Input: part model. Units: mm. Frame: model coordinates. Round coordinates to 2 decimals unless told otherwise and drop trailing zeros. Loops run counter-clockwise (first coordinate to the right, second up) from the corner with the lowest first, then second, coordinate; pieces in that order, holes last. Notation, with made-up numbers: (-1, 84.5) - (42, 84.5) arc R7 ccw to (42, 92.5) - close; hole circle Ø6 at (10, 51). An arc over 180 degrees is marked (long way). Write each question's results on one line, items separated by ' | '.
from build123d import *

# Parameters (mm, degrees)
F1_DEPTH    = 3
F2_DEPTH    = 25
F3_R        = 20
F4_R        = 100
F5_T1_DEPTH = 28.2643660281


# Not quite as in the source:
# - a fillet or chamfer that OpenCascade refuses, or shapes differently, is made with other operations: its cross-section is extruded or revolved along the edge and cut away or added


with BuildPart() as f1:
    # F0 (on Front) → F1 (new body)
    with BuildSketch(Plane.XZ):
        with BuildLine():
            ThreePointArc((-119.2295857728, 16.5976797057), (-89.2269882152, -21.8866064143), (-44.5863344816, -2.1785326218))
            ThreePointArc((-44.5863344816, -2.1785326218), (-31.5003837254, 22.7075657451), (-18.8527258188, 47.819251244))
            ThreePointArc((-18.8527258188, 47.819251244), (-11.5073907558, 58.7139707042), (-8.9261215756, 71.5975225718))
            Line((-8.9261215756, 71.5975225718), (-11.67442069, 71.5975225718))
            Line((-11.67442069, 71.5975225718), (-11.67442069, 74.0203762137))
            ThreePointArc((-11.67442069, 74.0203762137), (-12.7707106261, 77.9833199576), (-14.3762885703, 81.7686725444))
            ThreePointArc((-14.3762885703, 81.7686725444), (-44.33377908, 98.9465167224), (-71.9061774941, 78.1548738354))
            Line((-71.9061774941, 78.1548738354), (-107.2845857728, 78.1548738354))
            Line((-107.2845857728, 78.1548738354), (-119.2295857728, 78.1548738354))
            Line((-119.2295857728, 78.1548738354), (-119.2295857728, 66.2098738354))
            Line((-119.2295857728, 66.2098738354), (-119.2295857728, 16.5976797057))
        make_face()
        with BuildLine():
            ThreePointArc((-26.6928125913, 79.0930187933), (-24.6315082315, 75.5227380173), (-23.3711215756, 71.597523888))
            Line((-23.3711215756, 71.597523888), (-20.8711215756, 71.5975236602))
            ThreePointArc((-20.8711215756, 71.5975236602), (-22.8939959961, 62.4935676044), (-28.5819229469, 55.1029300277))
            ThreePointArc((-28.5819229469, 55.1029300277), (-41.6104278008, 29.1671780434), (-55.1096433175, 3.4732809051))
            ThreePointArc((-55.1096433175, 3.4732809051), (-86.3130475025, -10.3024804429), (-107.2845857728, 16.5976797057))
            Line((-107.2845857728, 16.5976797057), (-107.2845857728, 66.2098738354))
            Line((-107.2845857728, 66.2098738354), (-104.7845857728, 66.2098738354))
            Line((-104.7845857728, 66.2098738354), (-68.5864427672, 66.2098738354))
            Line((-68.5864427672, 66.2098738354), (-63.1803487139, 66.2098738354))
            ThreePointArc((-63.1803487139, 66.2098738354), (-63.6941147242, 68.8812286524), (-63.8664115811, 71.5960777945))
            Line((-63.8664115811, 71.5960777945), (-61.3664115868, 71.5962461647))
            ThreePointArc((-61.3664115868, 71.5962461647), (-46.4685424734, 86.625019162), (-26.6928125913, 79.0930187933))
        make_face(mode=Mode.SUBTRACT)
        with BuildLine():
            ThreePointArc((-32.7025071715, 52.3956462756), (-51.243606048, 52.0172813271), (-63.1803487139, 66.2098738354))
            Line((-63.1803487139, 66.2098738354), (-68.5864427672, 66.2098738354))
            Line((-68.5864427672, 66.2098738354), (-104.7845857728, 66.2098738354))
            Line((-104.7845857728, 66.2098738354), (-104.7845857728, 16.5976797057))
            ThreePointArc((-104.7845857728, 16.5976797057), (-85.7031813006, -7.8780087034), (-57.3120938901, 4.6561636023))
            ThreePointArc((-57.3120938901, 4.6561636023), (-44.8056231456, 28.4219407394), (-32.7025071715, 52.3956462756))
        make_face()
        with BuildLine():
            ThreePointArc((-61.3664115868, 71.5962461647), (-42.368127741, 52.5998806027), (-23.3711215756, 71.597523888))
            Line((-23.3711215756, 71.597523888), (-28.5062876117, 71.7030383349))
            ThreePointArc((-28.5062876117, 71.7030383348), (-35.0280474509, 67.9936357913), (-42.4162418184, 66.6868830916))
            ThreePointArc((-42.4162418184, 66.6868830916), (-49.8149115034, 67.9342855665), (-56.3664115866, 71.5913571683))
            Line((-56.3664115866, 71.5913571683), (-61.3664115868, 71.5962461647))
        make_face()
        with BuildLine():
            ThreePointArc((-55.1096433175, 3.4732809051), (-41.6104278008, 29.1671780434), (-28.5819229469, 55.1029300277))
            ThreePointArc((-28.5819229469, 55.1029300277), (-30.5643455059, 53.6307678626), (-32.7025071715, 52.3956462756))
            ThreePointArc((-32.7025071715, 52.3956462756), (-44.8056231456, 28.4219407394), (-57.3120938901, 4.6561636023))
            ThreePointArc((-57.3120938901, 4.6561636023), (-85.7031813006, -7.8780087034), (-104.7845857728, 16.5976797057))
            Line((-104.7845857728, 16.5976797057), (-104.7845857728, 66.2098738354))
            Line((-104.7845857728, 66.2098738354), (-107.2845857728, 66.2098738354))
            Line((-107.2845857728, 66.2098738354), (-107.2845857728, 16.5976797057))
            ThreePointArc((-107.2845857728, 16.5976797057), (-86.3130475025, -10.3024804429), (-55.1096433175, 3.4732809051))
        make_face()
        with BuildLine():
            ThreePointArc((-42.4162418184, 66.6868830916), (-35.0280474509, 67.9936357913), (-28.5062876117, 71.7030383348))
            ThreePointArc((-28.5062876117, 71.7030383349), (-42.4756351565, 81.447422187), (-56.3664115866, 71.5913571683))
            ThreePointArc((-56.3664115866, 71.5913571683), (-49.8149115034, 67.9342855665), (-42.4162418184, 66.6868830916))
        make_face()
        with BuildLine():
            Line((-28.5062876117, 71.7030383349), (-23.3711215756, 71.597523888))
            ThreePointArc((-23.3711215756, 71.597523888), (-24.6315082315, 75.5227380173), (-26.6928125913, 79.0930187933))
            ThreePointArc((-26.6928125913, 79.0930187933), (-46.4685424734, 86.625019162), (-61.3664115868, 71.5962461647))
            Line((-61.3664115868, 71.5962461647), (-56.3664115866, 71.5913571683))
            ThreePointArc((-56.3664115866, 71.5913571683), (-42.4756351565, 81.447422187), (-28.5062876117, 71.7030383349))
        make_face()
        with BuildLine():
            Line((-20.8711215756, 71.5975236602), (-23.3711215756, 71.597523888))
            ThreePointArc((-23.3711215756, 71.597523888), (-42.368127741, 52.5998806027), (-61.3664115868, 71.5962461647))
            Line((-61.3664115868, 71.5962461647), (-63.8664115811, 71.5960777945))
            ThreePointArc((-63.8664115811, 71.5960777945), (-63.6941147242, 68.8812286524), (-63.1803487139, 66.2098738354))
            ThreePointArc((-63.1803487139, 66.2098738354), (-51.243606048, 52.0172813271), (-32.7025071715, 52.3956462756))
            ThreePointArc((-32.7025071715, 52.3956462756), (-30.5643455059, 53.6307678626), (-28.5819229469, 55.1029300277))
            ThreePointArc((-28.5819229469, 55.1029300277), (-22.8939959961, 62.4935676044), (-20.8711215756, 71.5975236602))
        make_face()
    extrude(amount=F1_DEPTH)

    # F0 (on Front) → F2 (cut)
    with BuildSketch(Plane.XZ):
        with BuildLine():
            ThreePointArc((-42.4162418184, 66.6868830916), (-35.0280474509, 67.9936357913), (-28.5062876117, 71.7030383348))
            ThreePointArc((-28.5062876117, 71.7030383349), (-42.4756351565, 81.447422187), (-56.3664115866, 71.5913571683))
            ThreePointArc((-56.3664115866, 71.5913571683), (-49.8149115034, 67.9342855665), (-42.4162418184, 66.6868830916))
        make_face()
    extrude(amount=F2_DEPTH, mode=Mode.SUBTRACT)

    # F3
    f3_edges = [f1.edges().sort_by_distance(p)[0] for p in [
        (-119.229586, -1.5, 78.154874),
    ]]
    fillet(f3_edges, radius=F3_R)

    # F4
    f4_edges = [f1.edges().sort_by_distance(p)[0] for p in [
        (-71.906177, -1.5, 78.154874),
    ]]
    fillet(f4_edges, radius=F4_R)

    # F5: fillet of radius 5 on 1 edges, made by hand

    # F5_s2 → F5_t1 (cut)
    with BuildSketch(Plane.XZ.offset(-12.632183014)):
        with BuildLine():
            ThreePointArc((-11.67442069, 71.5975225718), (-9.7251397256, 69.4380959712), (-9.3078431517, 66.5590886613))
            ThreePointArc((-9.3078431517, 66.5590886613), (-9.0216886325, 69.0710859777), (-8.9261215756, 71.5975225718))
            Line((-8.9261215756, 71.5975225718), (-11.67442069, 71.5975225718))
        make_face()
    extrude(amount=F5_T1_DEPTH, mode=Mode.SUBTRACT)


solid = f1.part
1. Line query: line 1 (Z direction, x = -38.5, y = -0.65); line 2 (Z direction, x = -37, y = -1.15) (3 decimals); line 3 (Z direction, x = -109.5, y = -0.75). Output: solid intervals per line, ascending. Write a range as [from, to].
Answer:
line 1: [9.26, 67.05], [80.92, 98.77] | line 2: [12.119, 67.385], [80.421, 98.545] | line 3: [-9.43, 75.32]
2. Mould query, pull axis Z, two halves, no side actions, for faces 1 (the cylindrical face through (-9.743, -1.479, 69.475)), 2 (the cylindrical face through (-31.68, -1.48, 22.36)), 3 (the flat face through (-65, -3, 39)), 4 (the cylindrical face through (-42.222, -1.479, 81.446)). Classes: pulls with the +Z half, pulls with the -Z half, needs draft (parallel to the pull), parting line crosses it, or undercut.
Answer:
face 1: parting line crosses it | face 2: pulls with the -Z half | face 3: needs draft | face 4: undercut
3. Contact query for flat-ended pins moving along their axis: pin 1 (1 mm diameter, centred on x = -98, y = -2.5, fed in from -Z); pin 2 (1.5 mm diameter, centred on y = -2.5, z = 12.5, fed in from -X). Output: stop coordinate, or through.
Answer:
pin 1: z = -18.79 | pin 2: x = -119.09
4. Section query B-B, the plane z = 26.5. Output: boundary loops of the cut face in (x, y), plus the area to 3 significant figures.
Answer:
outline: (-119.23, -3) - (-29.55, -3) - (-29.55, 0) - (-119.23, 0) - close | area: 269 mm^2
5. Section query C-C, the plane x = -109. Output: boundary loops of the cut face in (y, z).
Answer:
outline: (-3, -10) - (0, -10) - (0, 75.61) - (-3, 75.61) - close
6. Section query A-A, the plane x = -31.5. Output: boundary loops of the cut face in (y, z), plus the area to 3 significant figures.
Answer:
outline: (-3, 22.71) - (0, 22.71) - (0, 69.63) - (-3, 69.63) - close; (-3, 76.64) - (0, 76.64) - (0, 97.06) - (-3, 97.06) - close | area: 202 mm^2
